```python
from build123d import *

# Parameters (mm, degrees)
SKETCH2_W               = 75
SKETCH2_H               = 60
BODY_CREATION_DEPTH     = 27
THIKNESS_OF_WALLS_T     = -1.5
SKETCH6_W               = 5.5
SKETCH6_H               = 5.5
CORNER_RECT_DEPTH       = 10
SKETCH8_R               = 1.2
SCREW_HOLE_DEPTH        = 27
SKETCH10_R              = 2
SCREW_HEAD_DEPTH        = 4
SKETCH5_W               = 9
SKETCH5_H               = 20.9
PORTS_CUT_OUT_DEPTH     = 1.5
SKETCH11_W              = 44.5
SKETCH11_H              = 1
SKETCH11_W_2            = 50
SKETCH11_W_3            = 1.25
SKETCH11_H_2            = 22.5
BATTERY_PLACEMENT_DEPTH = 10
FILLET1_R               = 1.5
FILLET2_R               = 2.93
SKETCH13_W              = 50
SKETCH13_H              = 40
CUT_EXTRUDE1_DEPTH      = 1


with BuildPart() as part:
    # Sketch2 → Body creation (new body)
    with BuildSketch(Plane.XY):
        with Locations((37.5, 30)):
            Rectangle(SKETCH2_W, SKETCH2_H)
    extrude(amount=BODY_CREATION_DEPTH)

    # Thikness of walls
    thikness_of_walls_openings = [part.faces().sort_by_distance(p)[0] for p in [
        (37.5, 30, 27),
    ]]
    offset(amount=THIKNESS_OF_WALLS_T, openings=thikness_of_walls_openings, kind=Kind.INTERSECTION)

    # Sketch6 → Corner rect. (add)
    with BuildSketch(Plane.XY.offset(1.5)):
        with Locations((4.25, 55.75)):
            Rectangle(SKETCH6_W, SKETCH6_H)
        with Locations((70.75, 55.75)):
            Rectangle(SKETCH6_W, SKETCH6_H)
    corner_rect = extrude(amount=CORNER_RECT_DEPTH)

    # Sketch8 → Screw hole (cut)
    with BuildSketch(Plane.XY.offset(27)):
        with Locations((4.35, 55.65)):
            Circle(SKETCH8_R)
        with Locations(Location((70.65, 55.65, 0), (0, 0, 180))):
            Circle(SKETCH8_R)
    screw_hole = extrude(amount=-SCREW_HOLE_DEPTH, mode=Mode.SUBTRACT)

    # Sketch10 → Screw head (cut)
    with BuildSketch(Plane(origin=(0, 0, 0), x_dir=(-1, 0, 0), z_dir=(0, 0, -1))):
        with Locations((-70.65, 55.65)):
            Circle(SKETCH10_R)
        with Locations((-4.35, 55.65)):
            Circle(SKETCH10_R)
    screw_head = extrude(amount=-SCREW_HEAD_DEPTH, mode=Mode.SUBTRACT)

    # Mirror to other side: Corner rect., Screw hole, Screw head across plane
    add(corner_rect.mirror(Plane(origin=(0, 30, 0), x_dir=(0, 0, 1), z_dir=(0, -1, 0))))
    add(screw_hole.mirror(Plane(origin=(0, 30, 0), x_dir=(0, 0, 1), z_dir=(0, -1, 0))), mode=Mode.SUBTRACT)
    add(screw_head.mirror(Plane(origin=(0, 30, 0), x_dir=(0, 0, 1), z_dir=(0, -1, 0))), mode=Mode.SUBTRACT)

    # Sketch5 → Ports cut out (cut)
    with BuildSketch(Plane.XZ):
        with Locations((16, 16.55)):
            Rectangle(SKETCH5_W, SKETCH5_H)
        with BuildLine():
            Line((29.95, 13.6), (34.95, 13.6))
            ThreePointArc((34.95, 13.6), (36.576345597, 14.273654403), (37.25, 15.9))
            Line((37.25, 15.9), (37.25, 27))
            Line((37.25, 27), (27.65, 27))
            Line((27.65, 27), (27.65, 15.9))
            ThreePointArc((27.65, 15.9), (28.323654403, 14.273654403), (29.95, 13.6))
        make_face()
    extrude(amount=-PORTS_CUT_OUT_DEPTH, mode=Mode.SUBTRACT)

    # Sketch11 → Battery Placement (add)
    with BuildSketch(Plane.XY.offset(1.5)):
        with Locations((29.25, 53.5)):
            Rectangle(SKETCH11_W, SKETCH11_H)
        with Locations((26.5, 16.8)):
            Rectangle(SKETCH11_W_2, SKETCH11_H)
        with Locations((67.375, 47.25)):
            Rectangle(SKETCH11_W_3, SKETCH11_H_2)
    extrude(amount=BATTERY_PLACEMENT_DEPTH)

    # Fillet1
    fillet1_edges = [part.edges().sort_by_distance(p)[0] for p in [
        (7, 56.25, 1.5),
        (51.5, 53.5, 1.5),
        (29.25, 54, 1.5),
        (1.5, 11.65, 1.5),
        (51.5, 16.8, 1.5),
        (26.5, 17.3, 1.5),
        (26.5, 16.3, 1.5),
        (36.875, 58.5, 1.5),
        (68, 44.5, 1.5),
        (66.75, 47.25, 1.5),
        (67.375, 36, 1.5),
        (1.5, 35.15, 1.5),
        (26.5, 53, 1.5),
        (70.75, 53, 1.5),
        (37.5, 1.5, 1.5),
        (4.25, 7, 1.5),
        (7, 4.25, 1.5),
        (73.5, 30, 1.5),
        (68, 4.25, 1.5),
        (70.75, 7, 1.5),
    ]]
    fillet(fillet1_edges, radius=FILLET1_R)

    # Fillet2
    # the kernel refuses this fillet: 2.93 mm, written as the material it takes off along each edge
    with BuildSketch(Plane(origin=(72.07, 57.07, 2.93), x_dir=(1, 0, 0), z_dir=(0, 1, 0))) as fillet2_piece_1_section:
        Polygon((0, 0), (FILLET2_R, 0), (FILLET2_R, FILLET2_R), (0, FILLET2_R), align=None)
    fillet2_piece_1 = extrude(amount=FILLET2_R, mode=Mode.PRIVATE)
    fillet2_piece_1 = fillet2_piece_1 - Plane(origin=(72.07, 57.07, 2.93), x_dir=(-0.7071067811865475, 0, 0.7071067811865475), z_dir=(0, 1, 0)) * Sphere(FILLET2_R, mode=Mode.PRIVATE)
    add(fillet2_piece_1, mode=Mode.SUBTRACT)
    with BuildSketch(Plane(origin=(2.93, 57.07, 2.93), x_dir=(0, 1, 0), z_dir=(-1, 0, 0))) as fillet2_piece_2_section:
        Polygon((0, 0), (FILLET2_R, 0), (FILLET2_R, FILLET2_R), (0, FILLET2_R), align=None)
    fillet2_piece_2 = extrude(amount=FILLET2_R, mode=Mode.PRIVATE)
    fillet2_piece_2 = fillet2_piece_2 - Plane(origin=(2.93, 57.07, 2.93), x_dir=(0, -0.7071067811865475, 0.7071067811865475), z_dir=(-1, 0, 0)) * Sphere(FILLET2_R, mode=Mode.PRIVATE)
    add(fillet2_piece_2, mode=Mode.SUBTRACT)
    with BuildSketch(Plane(origin=(72.07, 2.93, 2.93), x_dir=(0, -1, 0), z_dir=(1, 0, 0))) as fillet2_piece_3_section:
        Polygon((0, 0), (FILLET2_R, 0), (FILLET2_R, FILLET2_R), (0, FILLET2_R), align=None)
    fillet2_piece_3 = extrude(amount=FILLET2_R, mode=Mode.PRIVATE)
    fillet2_piece_3 = fillet2_piece_3 - Plane(origin=(72.07, 2.93, 2.93), x_dir=(0, 0.7071067811865475, 0.7071067811865475), z_dir=(1, 0, 0)) * Sphere(FILLET2_R, mode=Mode.PRIVATE)
    add(fillet2_piece_3, mode=Mode.SUBTRACT)
    with BuildSketch(Plane(origin=(2.93, 2.93, 2.93), x_dir=(0, -1, 0), z_dir=(-1, 0, 0))) as fillet2_piece_4_section:
        Polygon((0, 0), (FILLET2_R, 0), (FILLET2_R, -FILLET2_R), (0, -FILLET2_R), align=None)
    fillet2_piece_4 = extrude(amount=FILLET2_R, mode=Mode.PRIVATE)
    fillet2_piece_4 = fillet2_piece_4 - Plane(origin=(2.93, 2.93, 2.93), x_dir=(0, 0.7071067811865475, 0.7071067811865475), z_dir=(-1, 0, 0)) * Sphere(FILLET2_R, mode=Mode.PRIVATE)
    add(fillet2_piece_4, mode=Mode.SUBTRACT)
    with BuildSketch(Plane(origin=(72.07, 60, 0), x_dir=(0, 0, 1), z_dir=(-1, 0, 0)), Plane(origin=(2.93, 0, 0), x_dir=(0, 0, 1), z_dir=(1, 0, 0))) as fillet2_piece_5:
        with BuildLine():
            CenterArc((FILLET2_R, -FILLET2_R), FILLET2_R, 90, 90)
            Line((0, -FILLET2_R), (0, 0))
            Line((0, 0), (FILLET2_R, 0))
        make_face()
    extrude(amount=69.14, mode=Mode.SUBTRACT)
    with BuildSketch(Plane(origin=(75, 2.93, 0), x_dir=(0, 0, 1), z_dir=(0, 1, 0)), Plane(origin=(0, 57.07, 0), x_dir=(0, 0, 1), z_dir=(0, -1, 0))) as fillet2_piece_6:
        with BuildLine():
            CenterArc((FILLET2_R, -FILLET2_R), FILLET2_R, 90, 90)
            Line((0, -FILLET2_R), (0, 0))
            Line((0, 0), (FILLET2_R, 0))
        make_face()
    extrude(amount=54.14, mode=Mode.SUBTRACT)
    with BuildSketch(Plane(origin=(0, 60, 2.93), x_dir=(0, -1, 0), z_dir=(0, 0, 1)), Plane(origin=(75, 60, 2.93), x_dir=(-1, 0, 0), z_dir=(0, 0, 1)), Plane(origin=(75, 0, 2.93), x_dir=(0, 1, 0), z_dir=(0, 0, 1))) as fillet2_piece_7:
        with BuildLine():
            CenterArc((FILLET2_R, FILLET2_R), FILLET2_R, 180, 90)
            Line((0, FILLET2_R), (0, 0))
            Line((0, 0), (FILLET2_R, 0))
        make_face()
    extrude(amount=31.395, mode=Mode.SUBTRACT)
    with BuildSketch(Plane(origin=(0, 0, 2.93), x_dir=(0, 1, 0), z_dir=(0, 0, 1))) as fillet2_piece_8:
        with BuildLine():
            CenterArc((FILLET2_R, -FILLET2_R), FILLET2_R, 90, 90)
            Line((0, -FILLET2_R), (0, 0))
            Line((0, 0), (FILLET2_R, 0))
        make_face()
    extrude(amount=31.395, mode=Mode.SUBTRACT)

    # Sketch13 → Cut-Extrude1 (cut)
    with BuildSketch(Plane(origin=(0, 0, 0), x_dir=(-1, 0, 0), z_dir=(0, 0, -1))):
        with Locations((-37.5, 30)):
            Rectangle(SKETCH13_W, SKETCH13_H)
    extrude(amount=-CUT_EXTRUDE1_DEPTH, mode=Mode.SUBTRACT)


solid = part.part
```
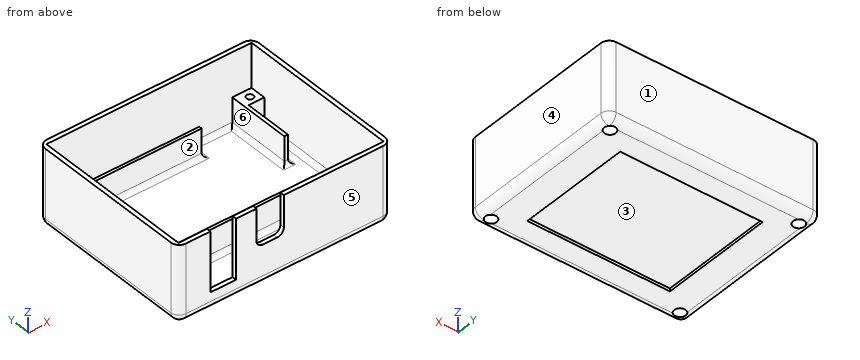
Can you work these out from the model? Positions are in its coordinate system, mm. Face numbers are marked on the shaded views. A direction names the side the tool comes from. Coordinates: 2 decimals unless noted, no trailing zeros. Loops run counter-clockwise (first coordinate to the right, second up) from the corner with the lowest first, then second, coordinate; pieces in that order, holes last. Notation, with made-up numbers: (12, -29) - (21, -29) arc R20 cw to (21, -10) - close; hole circle Ø7 at (50.25, 13). An arc over 180 degrees is marked (long way). Answer as CSV lines item,"result". Start each with the question number.
1) Which directions (+Z, -Z, +X, -X, +Y, -Y) give clear straight access to the entire face, cutting with the end or side of a thin tool? Please do the marked faces 1, 2 and 3.
2) Suppose I cut it at C-C (x = 47). Please give me the cut outline in (y, z), plus the area to 3 significant figures.
3) Suppose I cut it at B-B (y = 4.35). Count the separate pieces of the cut face and the enclosed holes in it, plus the area to 3 significant figures.
4) Suppose I cut it at A-A (z = 20.75). Please give me the cut outline in (x, y), plus the area to 3 significant figures.
5) I need wall thicknesses on line 1 (Y direction, x = 28, z = 11); line 2 (Y direction, x = 24, z = 24.5); line 3 (X direction, y = 51.5, z = 15.75). Which ranges of each line are inside material? Lowest first, please. Write a range as from..to.
6) Thinking about a two-plate mould opening in Y: for the marked faces 4, 5 and 6, which applies, pulls with the +Y half, pulls with the -Y half, needs draft (parallel to the pull), parting line crosses it, or undercut?
7) For pin 1 (1.4 mm diameter, centred on x = 4.35, y = 55.65, fed in from -Z); pin 2 (0.8 mm diameter, centred on x = 37.5, z = 0.5, fed in from +Y); pin 3 (1 mm diameter, centred on x = 54.5, y = 50, fed in from +Z); pin 4 (5 mm diameter, centred on x = 28.5, y = 30, fed in from -Z), each with a flat end and sliding along its axis, tell me the tip position at first contact or that it passes through.
Check result:
1,face 1,"+Z, -Z, +X, -X, +Y"
1,face 2,"+Z"
1,face 3,"-Z"
2,outline,"(0, 2.93) arc R2.93 ccw to (2.93, 0) - (10, 0) - (10, 1) - (50, 1) - (50, 0) - (57.07, 0) arc R2.93 ccw to (60, 2.93) - (60, 27) - (58.5, 27) - (58.5, 3) arc R1.5 cw to (57, 1.5) - (55.5, 1.5) arc R1.5 cw to (54, 3) - (54, 11.5) - (53, 11.5) - (53, 3) arc R1.5 cw to (51.5, 1.5) - (18.8, 1.5) arc R1.5 cw to (17.3, 3) - (17.3, 11.5) - (16.3, 11.5) - (16.3, 3) arc R1.5 cw to (14.8, 1.5) - (3, 1.5) arc R1.5 cw to (1.5, 3) - (1.5, 27) - (0, 27) - close"
2,area,"146 mm²"
3,separate pieces,"3"
3,enclosed holes,"0"
3,area,"228 mm²"
4,outline,"(0, 2.93) arc R2.93 ccw to (2.93, 0) - (11.5, 0) - (11.5, 1.5) - (1.5, 1.5) - (1.5, 58.5) - (73.5, 58.5) - (73.5, 1.5) - (37.25, 1.5) - (37.25, 0) - (72.07, 0) arc R2.93 ccw to (75, 2.93) - (75, 57.07) arc R2.93 ccw to (72.07, 60) - (2.93, 60) arc R2.93 ccw to (0, 57.07) - close; (20.5, 0) - (27.65, 0) - (27.65, 1.5) - (20.5, 1.5) - close"
4,area,"361 mm²"
5,line 1,"y = 0..1.5, 16.3..17.3, 53..54, 58.5..60"
5,line 2,"y = 0..1.5, 58.5..60"
5,line 3,"x = 0..1.5, 73.5..75"
6,face 4,"needs draft"
6,face 5,"pulls with the -Y half"
6,face 6,"undercut"
7,pin 1,"passes through"
7,pin 2,"stops at y = 59.18"
7,pin 3,"stops at z = 1.5"
7,pin 4,"stops at z = 1"
